For this review, take the finished solid that the model builds, in its own axes (mm). Face numbers are marked on the shaded views. A direction names the side the tool comes from. Give positions to 0.01 mm unless a question says otherwise; leave off trailing zeros. Loops run counter-clockwise (first coordinate to the right, second up) from the corner with the lowest first, then second, coordinate; pieces in that order, holes last. Notation, with made-up numbers: (-14, 83.25) - (38, 83.25) arc R25 cw to (38, 101.25) - close; hole circle Ø2 at (37, -14.5). An arc over 180 degrees is marked (long way). Put each result on its own line as item: value.
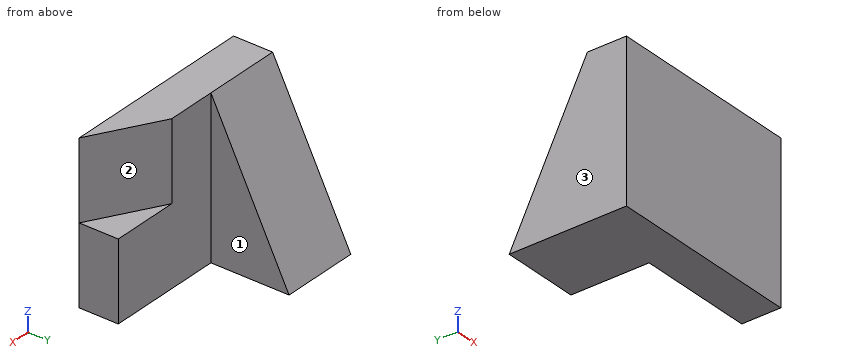
from build123d import *

# Parameters (mm, degrees)
SKETCH1_W           = 50
SKETCH1_H           = 40
BOSS_EXTRUDE1_DEPTH = 10
CUT_EXTRUDE1_DEPTH  = 20
SKETCH3_W           = 20
SKETCH3_H           = 40
BOSS_EXTRUDE2_DEPTH = 20
CUT_EXTRUDE2_DEPTH  = 20


with BuildPart() as part:
    # Sketch1 → Boss-Extrude1 (new body)
    with BuildSketch(Plane(origin=(0, 0, 0), x_dir=(1, 0, 0), z_dir=(0, 1, 0))):
        Rectangle(SKETCH1_W, SKETCH1_H)
    extrude(amount=BOSS_EXTRUDE1_DEPTH)

    # Sketch2 → Cut-Extrude1 (cut)
    with BuildSketch(Plane.XY.offset(20)):
        Polygon((25, 0), (7.679491924, 10), (25, 10), align=None)
    extrude(amount=-CUT_EXTRUDE1_DEPTH, mode=Mode.SUBTRACT)

    # Sketch3 → Boss-Extrude2 (add)
    with BuildSketch(Plane(origin=(0, 10, 0), x_dir=(1, 0, 0), z_dir=(0, 1, 0))):
        with Locations((-15, 0)):
            Rectangle(SKETCH3_W, SKETCH3_H)
    extrude(amount=BOSS_EXTRUDE2_DEPTH)

    # Sketch4 → Cut-Extrude2 (cut)
    with BuildSketch(Plane(origin=(-5, 0, 0), x_dir=(0, 0, -1), z_dir=(1, 0, 0))):
        Polygon((20, 30), (-20, 10), (-20, 30), align=None)
    extrude(amount=-CUT_EXTRUDE2_DEPTH, mode=Mode.SUBTRACT)


solid = part.part
1) Take a section at B-B on y = 12.5. State the section outline as (x, z) points.
Geometry check:
outline: (-25, -20) - (-5, -20) - (-5, 15) - (-25, 15) - close
2) Take a section at C-C on x = 6. State the section outline as (y, z) points, and give its area (3 significant figures).
Geometry check:
outline: (0, -20) - (10, -20) - (10, 20) - (0, 20) - close
area: 400 mm²
3) For the marked faces 1, 2 and 3, list the 3-axis set-ups (+Z, -Z, +X, -X, +Y, -Y) from which the entire face can be reached by the end or side of a thin tool; tool diameter is ignored.
Geometry check:
face 1: +Z, -Z, +X, +Y
face 2: +Z, +X, +Y
face 3: +Z, -Z, -X, +Y, -Y
4) Wall thickness on line 1 (Y direction, x = 0, z = 12); line 2 (X direction, y = 12.5, z = 10); line 3 (Z direction, x = 18.5, y = 5.5): over which ranges is each line inside the solid? List them lowest first.
Geometry check:
line 1: y = 0 to 10
line 2: x = -25 to -5
line 3: z = -20 to 0
5) Take a section at D-D on z = -11. State the section outline as (x, y) points.
Geometry check:
outline: (-25, 0) - (25, 0) - (25, 10) - (-5, 10) - (-5, 25.5) - (-25, 25.5) - close
6) Take a section at A-A on z = 3.5. State the section outline as (x, y) points, and give its area (3 significant figures).
Geometry check:
outline: (-25, 0) - (25, 0) - (7.68, 10) - (-5, 10) - (-5, 18.25) - (-25, 18.25) - close
area: 578 mm²
7) Insertion check: pin 1 Ø5 at (x, y) = (-13, 19) entering from +Z. The pin has a flat end and moves straight along its axis. Give the tip position at first contact, or say it passes through.
Geometry check:
pin 1: stops at z = 7
